For this review, use the dimensioned drawing (mm, ordinates from the lowest corner) and the shaded views. Coordinates: 2 decimals unless noted, no trailing zeros. Order: outer loops, then holes, each group sorted by start corner. A loop starts at its lowest first (then second) coordinate and runs counter-clockwise, first axis right, second up. Notation, with made-up numbers: M -22.5,27 L 14.5,27 A13 ccw 14.5,39 Z; hole C 50.5,8.5 d11. An arc over 180 degrees is marked long. One line per item, written item: value.
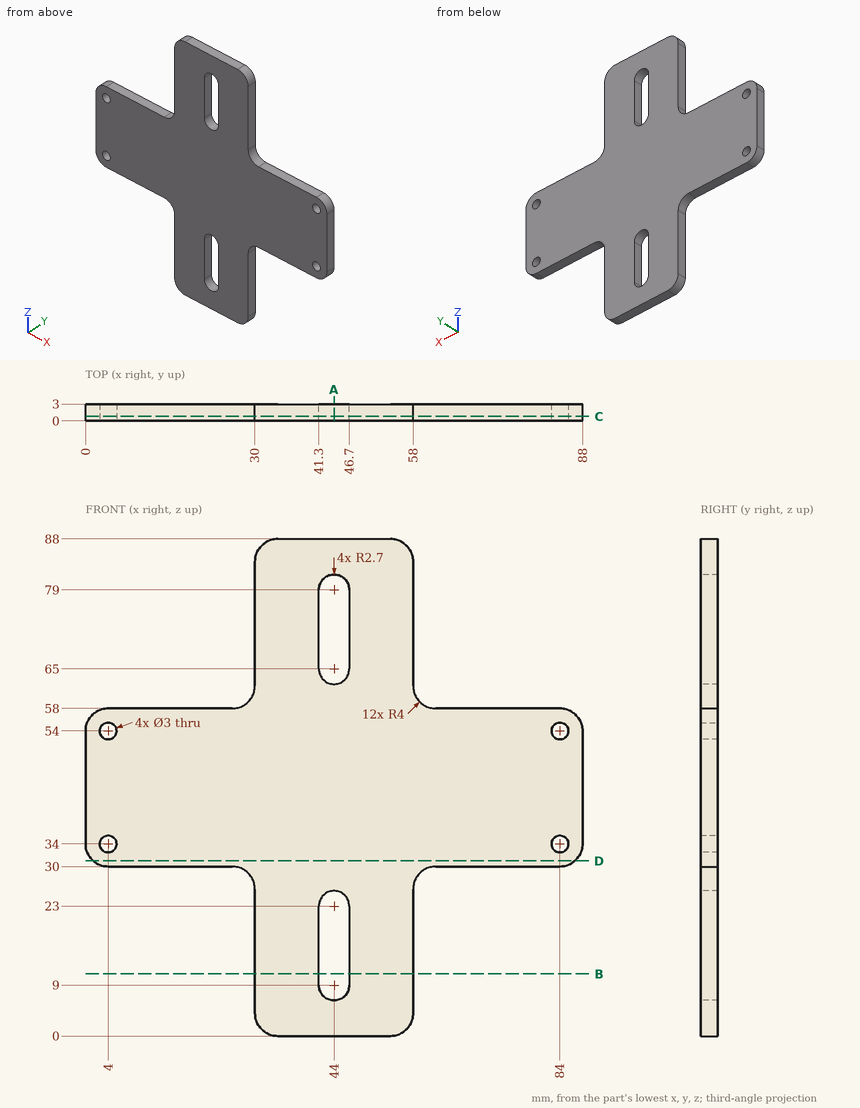
(1) For L1, parallel to Z at x = 4, y = 1.85; L2, parallel to X at y = 0.75, z = 54; L3, parallel to X at y = 2.2, z = 75.5, list the stretches that pass through material, from the lowest coordinate up.
Geometry results:
L1: z = 30 to 32.5, 35.5 to 52.5, 55.5 to 58
L2: x = 0 to 2.5, 5.5 to 82.5, 85.5 to 88
L3: x = 30 to 41.3, 46.7 to 58
(2) We need section B-B, the plane z = 11. State the section outline as (x, y) points, plus the area to 3 significant figures.
Geometry results:
outline: M 30,0 L 41.3,0 L 41.3,3 L 30,3 Z; M 46.7,0 L 58,0 L 58,3 L 46.7,3 Z
area: 67.8 mm2
(3) We need section D-D, the plane z = 31. State the section outline as (x, y) points, plus the area to 3 significant figures.
Geometry results:
outline: M 1.35,0 L 86.65,0 L 86.65,3 L 1.35,3 Z
area: 256 mm2
(4) We need section A-A, the plane x = 44. State the section outline as (y, z) points, plus the area to 3 significant figures.
Geometry results:
outline: M 0,0 L 3,0 L 3,6.3 L 0,6.3 Z; M 0,25.7 L 3,25.7 L 3,62.3 L 0,62.3 Z; M 0,81.7 L 3,81.7 L 3,88 L 0,88 Z
area: 148 mm2
(5) We need section C-C, the plane y = 0.8. Count the separate pieces of the cut face and the enclosed holes in it, plus the area to 3 significant figures.
Geometry results:
separate pieces: 1
enclosed holes: 6
area: 3,900 mm2
(6) Insertion check: pin 1 Ø1 at (y, z) = (0.5, 65) entering from +X; pin 2 Ø1 at (x, y) = (24.5, 2) entering from +Z; pin 3 Ø2.5 at (x, z) = (4, 54) entering from +Y; pin 4 Ø1.5 at (x, y) = (21, 2.5) entering from -Z. Each pin has a flat end and moves straight along its axis. Give the tip position at first contact, or say it passes through.
Geometry results:
pin 1: stops at x = 58
pin 2: stops at z = 58
pin 3: passes through
pin 4: stops at z = 30
